Autodesk Inventor part; units mm, degrees
ref_plane "YZ Plane" through (0, 0, 0) normal (1, 0, 0) x (0, 1, 0)
ref_plane "XZ Plane" through (0, 0, 0) normal (0, 1, 0) x (-1, 0, 0)
ref_plane "XY Plane" through (0, 0, 0) normal (0, 0, 1) x (1, 0, 0)
sketch "Sketch1" plane through (0, 0, 0) normal (1, 0, 0) x (0, 1, 0)
  line L0 (0, 13.75) -> (-5.2, 13.75)
  line L1 (-5.2, 13.75) -> (-5.2, 6.2)
  line L2 (-5.2, 6.2) -> (-7.4, 6.2)
  line L3 (-7.4, 6.2) -> (-7.4, 2.5)
  line L4 (-7.4, 2.5) -> (-13.4, 2.5) construction
  line L5 (-13.4, 2.5) -> (-13.4, -1.6142) construction
  line L6 (-16.08, 0) -> (2.68, 0) construction
  line L7 (0, -13.75) -> (-5.2, -13.75)
  line L8 (-5.2, -13.75) -> (-5.2, -6.2)
  line L9 (-5.2, -6.2) -> (-7.4, -6.2)
  line L10 (-7.4, -6.2) -> (-7.4, -2.5)
  line L11 (-7.4, -2.5) -> (-13.4, -2.5) construction
  line L12 (-13.4, -2.5) -> (-13.4, -1.6142) construction
  line L13 (0, 13.75) -> (0, -13.75)
  line L14 (-7.4, 2.5) -> (-7.4, -2.5)
  point P0 (0, 0)
  dimension "d1" = 5
  dimension "d2" = 3.7
  dimension "d3" = 6
  dimension "d4" = 2.2
  dimension "d5" = 5.2
  dimension "d52" = 27.5
  dimension "d53" = 7.55
extrude "Extrusion1" add sketch "Sketch1" along normal blind 22
sketch "Sketch2" plane through (0, -5.2, -13.75) normal (0, 0, -1) x (-1, 0, 0)
  line L0 (0, 0) -> (0, 5.2)
  line L1 (0, 5.2) -> (-22, 5.2)
  line L2 (-22, 0) -> (-22, 5.2)
  line L3 (0, 0) -> (-22, 0)
  point P0 (0, 5.2)
extrude "Extrusion2" add sketch "Sketch2" along normal blind 14
sketch "Sketch3" plane through (0, 0, 13.75) normal (0, 1, 0) x (1, 0, 0)
  circle A0 centre (3.3, 22.5) radius 1.3 construction
  circle A1 centre (8.9569, 28.1569) radius 1.55 construction
  line L0 (3.3, 22.5) -> (8.9569, 28.1569) construction
  line L1 (8.9569, 28.1569) -> (2.1344, 28.1569) construction
  line L2 (0, 0) -> (22, 0) construction
  line L3 (22, 41.5) -> (0, 41.5) construction
  line L4 (3.3, 22.5) -> (3.3, 32.5) construction
  line L5 (8.9569, 28.1569) -> (8.9569, 38.1569) construction
  line L6 (0, 0) -> (0, 41.5)
  point P0 (0, 13.75)
  point P1 (6.1284, 25.3284)
  point P2 (3.3, 27.5)
  point P3 (0, 19.95)
  point P4 (0, 27.5)
  point P5 (0, 27.5)
  point P6 (0, 27.5)
  dimension "d10" = 2.6
  dimension "d11" = 3.1
  dimension "d12" = 45
  dimension "d17" = 5
  dimension "d43" = 3.3
  dimension "d44" = 8
  dimension "d46" = 0
sketch "Sketch4" plane through (0, 0, 13.75) normal (0, 1, 0) x (1, 0, 0)
  line L0 (8.9569, 28.1569) -> (8.9569, 38.1569) construction
  line L1 (3.3, 22.5) -> (3.3, 32.5) construction
  line L2 (8.9569, 28.1569) -> (8.9569, 38.1569) construction
  line L3 (10.5069, 28.1569) -> (10.5069, 38.1569)
  line L4 (7.4069, 38.1569) -> (7.4069, 28.1569)
  arc A0 (7.4069, 28.1569) -> (10.5069, 28.1569) centre (8.9569, 28.1569) ccw
  arc A1 (10.5069, 38.1569) -> (7.4069, 38.1569) centre (8.9569, 38.1569) ccw
  circle A2 centre (8.9569, 28.1569) radius 1.55 construction
  circle A3 centre (3.3, 22.5) radius 1.3 construction
  line L5 (3.3, 22.5) -> (3.3, 32.5) construction
  line L6 (4.6, 22.5) -> (4.6, 32.5)
  line L7 (2, 32.5) -> (2, 22.5)
  arc A4 (2, 22.5) -> (4.6, 22.5) centre (3.3, 22.5) ccw
  arc A5 (4.6, 32.5) -> (2, 32.5) centre (3.3, 32.5) ccw
  point P0 (0, 13.75)
  point P1 (8.9569, 33.1569)
  point P2 (3.3, 27.5)
extrude "Extrusion3" cut sketch "Sketch4" against normal blind 3
sketch "Sketch5" plane through (0, 0, 13.75) normal (0, 1, 0) x (1, 0, 0)
  point P0 (0, 13.75)
ref_plane "Work Plane1" through (0, -2, 13.75) normal (0, 1, 0) x (1, 0, 0)
sketch "Sketch6" plane through (0, -2, 13.75) normal (0, 1, 0) x (1, 0, 0)
  line L0 (0.75, 23.9722) -> (3.3, 25.4445) construction
  line L1 (3.3, 25.4445) -> (5.85, 23.9722) construction
  line L2 (5.85, 23.9722) -> (5.85, 21.0278) construction
  line L3 (5.85, 21.0278) -> (3.3, 19.5555)
  line L4 (0.75, 21.0278) -> (0.75, 23.9722) construction
  line L5 (2, 22.5) -> (2, 32.5) construction
  line L6 (2, 27.5) -> (4.6, 27.5) construction
  line L7 (4.6, 32.5) -> (4.6, 22.5) construction
  line L8 (5.85, 33.9722) -> (3.3, 35.4445)
  line L9 (5.85, 21.0278) -> (5.85, 33.9722)
  line L10 (3.3, 19.5555) -> (0, 19.5555)
  line L11 (0, 7.55) -> (0, 19.95)
  line L12 (3.3, 35.4445) -> (0, 35.4445)
  line L13 (0, 0) -> (0, 41.5)
  line L14 (0, 19.5555) -> (0, 35.4445)
  point P0 (0, 13.75)
  point P1 (3.3, 22.5)
  point P2 (3.3, 22.5)
  point P3 (3.3, 27.5)
  point P4 (0, 11.25)
  dimension "d21" = 5.1
extrude "Extrusion4" cut sketch "Sketch6" against normal through all
sketch "Sketch7" plane through (0, 0, 13.75) normal (0, 1, 0) x (1, 0, 0)
  line L0 (32.7, 13.75) -> (-26.1, 13.75) construction
  circle A0 centre (15.8, 13.75) radius 4.5
  line L1 (22, 0) -> (22, 41.5)
  circle A1 centre (3.3, 22.5) radius 7 construction
  line L2 (0, 0) -> (22, 0) construction
  line L3 (10.3, 0) -> (10.3, 41.5) construction
  line L4 (22, 41.5) -> (0, 41.5) construction
  line L5 (11.3, 0) -> (11.3, 41.5) construction
  point P0 (0, 13.75)
  dimension "d24" = 9
  dimension "d39" = 14
  dimension "d41" = 1
hole "Hole1" at (15.8, 0, 0) direction (0, -1, 0) diameter 5.5 end through all counterbore diameter 10 counterbore depth 5
sketch "Sketch9" plane through (0, 0, 13.75) normal (0, 1, 0) x (1, 0, 0)
  line L0 (22, 19.95) -> (22, 41.5)
  line L1 (22, 27.5) -> (12.5069, 27.5)
  line L2 (12.5069, 27.5) -> (12.5069, 41.5)
  line L3 (12.5069, 41.5) -> (22, 41.5)
  line L4 (22, 41.5) -> (22, 27.5)
  line L5 (10.5069, 38.1569) -> (10.5069, 28.1569)
  line L6 (0, 41.5) -> (22, 41.5)
  point P0 (0, 13.75)
  point P1 (10.5069, 37.5)
  point P2 (0, 27.5)
  point P3 (0, 27.5)
  point P4 (0, 27.5)
  dimension "d45" = 2
extrude "Extrusion6" cut sketch "Sketch9" against normal through all
fillet "Fillet1" radius 2 1 edges at (12.5069, -2.6, -27.75)
fillet "Fillet2" radius 2 1 edges at (0, -2.6, -27.75)
sketch "Sketch10" plane through (0, 0, 13.75) normal (0, 1, 0) x (1, 0, 0)
  circle A0 centre (3.3, 22.5) radius 21 construction
  point P0 (0, 13.75)
  dimension "d51" = 42
properties part number "Dreiwegehahn_Montage45"
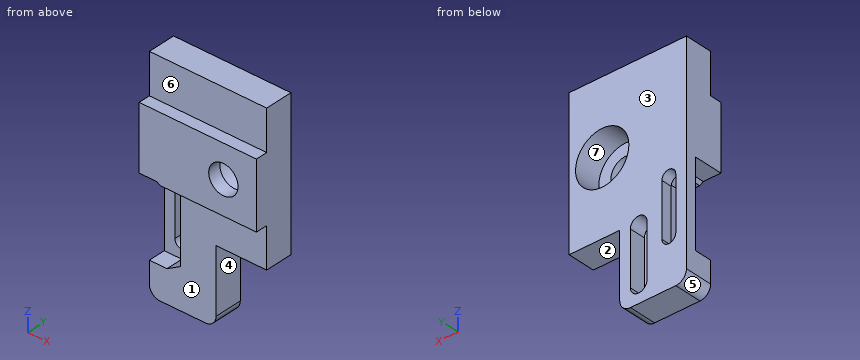
Here's how the part is built. I have some questions about the finished solid (model axes, mm). Face numbers are marked on the shaded views. A direction names the side the tool comes from. Coordinates: 2 decimals unless noted, no trailing zeros. Order: outer loops, then holes, each group sorted by start corner. A loop starts at its lowest first (then second) coordinate and runs counter-clockwise, first axis right, second up. Notation, with made-up numbers: (43, 28.25) -> (100, 28.25) arc R16 cw to (100, 33.25) -> close; hole circle Ø8 at (78.25, 26.5). An arc over 180 degrees is marked (long way). Return JSON: item names as keys, results as strings.
1) If I drill on probe 1 along X at (y, z) = (-1.3, 0); probe 2 along Z at (x, y) = (15.5, -3.25); probe 3 along Z at (x, y) = (15.8, -6.1), over which ranges is the centre line in solid material (lowest first)?
Conclusion:
{"probe 1": "x = 0 to 10.8, 20.8 to 22", "probe 2": "z = -13.75 to -4.99, 4.99 to 13.75", "probe 3": "z = -6.2 to -2.75, 2.75 to 6.2"}
2) If we section it at A-A on z = -12: List the corners of the cut face in (x, y) for me, plus the area to 3 significant figures.
Conclusion:
{"outline": "(0, -2) -> (2, -2) -> (2, 0) -> (0, 0) -> close; (4.6, -2) -> (5.85, -2) -> (5.85, -5.2) -> (22, -5.2) -> (22, 0) -> (4.6, 0) -> close", "area": "90.5 mm²"}
3) If we section it at B-B on y = -3.5: List the corners of the cut face in (x, z) for me, plus the area to 3 significant figures.
Conclusion:
{"outline": "(0, -25.75) arc R2 ccw to (2, -27.75) -> (10.51, -27.75) arc R2 ccw to (12.51, -25.75) -> (12.51, -13.75) -> (22, -13.75) -> (22, 13.75) -> (0, 13.75) -> (0, -5.81) -> (3.3, -5.81) -> (5.85, -7.28) -> (5.85, -20.22) -> (3.3, -21.69) -> (0, -21.69) -> close; hole circle Ø10 at (15.8, 0)", "area": "611 mm²"}
4) On a 3-axis mill with a long thin cutter (end or side, diameter ignored), from which of +Z, -Z, +X, -X, +Y, -Y can I reach the whole of each face in a straight line? I mean the marked faces 1, 2 and 3. Say none if no direction works.
Conclusion:
{"face 1": "-Z, +X, -X, -Y", "face 2": "-Z, +X, +Y, -Y", "face 3": "+Z, -Z, +X, -X, +Y"}
5) I'm going to push flat-ended pins straight in: P1, Ø2.5, axis at x = 10.5, z = 11.5, coming from the -Y side; P2, Ø1.5, axis at y = -1.5, z = -17.5, coming from the +X side; P3, Ø1.6, axis at y = -3, z = -16.5, coming from the -X side; P4, Ø1.5, axis at y = -6.5, z = -12, coming from the +X side. Where does each tip first touch, or does it pass through?
Conclusion:
{"P1": "stops at y = -5.2", "P2": "stops at x = 12.51", "P3": "stops at x = 5.85", "P4": "passes through"}
6) If we section it at D-D on z = 0: List the corners of the cut face in (x, y) for me, plus the area to 3 significant figures.
Conclusion:
{"outline": "(0, -7.4) -> (13.05, -7.4) -> (13.05, -5) -> (10.8, -5) -> (10.8, 0) -> (0, 0) -> close; (18.55, -7.4) -> (22, -7.4) -> (22, 0) -> (20.8, 0) -> (20.8, -5) -> (18.55, -5) -> close", "area": "99.6 mm²"}
7) Thinking about a two-plate mould opening in X: for the marked faces 4, 5, 6 and 7, which applies, +X half, -X half, draft (parallel to the pull), parting line (faces both ways), or undercut?
Conclusion:
{"face 4": "+X half", "face 5": "-X half", "face 6": "draft", "face 7": "undercut"}
8) If we section it at C-C on x = 15.8: List the corners of the cut face in (y, z) for me.
Conclusion:
{"outline": "(-7.4, -6.2) -> (-5.2, -6.2) -> (-5.2, -13.75) -> (0, -13.75) -> (0, -5) -> (-5, -5) -> (-5, -2.75) -> (-7.4, -2.75) -> close; (-7.4, 2.75) -> (-5, 2.75) -> (-5, 5) -> (0, 5) -> (0, 13.75) -> (-5.2, 13.75) -> (-5.2, 6.2) -> (-7.4, 6.2) -> close"}
